Part model, mm, in its own coordinate system. A direction names the side the tool comes from. Give positions to 0.01 mm unless a question says otherwise; leave off trailing zeros. Order: outer loops, then holes, each group sorted by start corner. A loop starts at its lowest first (then second) coordinate and runs counter-clockwise, first axis right, second up. Notation, with made-up numbers: (23.25, 57.25) - (52.25, 57.25) arc R19 cw to (52.25, 66.25) - close; hole circle Ø9 at (70.5, -36.75). An arc over 180 degrees is marked (long way). One line per item, written item: value.
```python
from build123d import *

# Parameters (mm, degrees)
BASE_FLANGIA1_DEPTH       = 477.5
BORDO_FLANGIA1_DEPTH      = 436
BORDO_FLANGIA1_BEND_DEPTH = 436
TAGLIO_ESTRUSIONE2_START  = -275
TAGLIO_ESTRUSIONE2_DEPTH  = 550


# Read off the part's stored shape, not the designer's step: Taglio-Estrusione2
# Sheet-metal steps are written as plain solids
with BuildPart() as part:
    # Schizzo1 → Base-Flangia1 (new, symmetric)
    with BuildSketch(Plane.XY):
        with BuildLine():
            Line((-255, 50), (-228, 50))
            ThreePointArc((-228, 50), (-225.878679656, 49.121320344), (-225, 47))
            Line((-225, 47), (-225, 7))
            ThreePointArc((-225, 7), (-222.949747468, 2.050252532), (-218, 0))
            Line((-218, 0), (218, 0))
            ThreePointArc((218, 0), (222.949747468, 2.050252532), (225, 7))
            Line((225, 7), (225, 47))
            ThreePointArc((225, 47), (225.878679656, 49.121320344), (228, 50))
            Line((228, 50), (255, 50))
            Line((255, 50), (255, 54))
            Line((255, 54), (228, 54))
            ThreePointArc((228, 54), (223.050252532, 51.949747468), (221, 47))
            Line((221, 47), (221, 7))
            ThreePointArc((221, 7), (220.121320344, 4.878679656), (218, 4))
            Line((218, 4), (-218, 4))
            ThreePointArc((-218, 4), (-220.121320344, 4.878679656), (-221, 7))
            Line((-221, 7), (-221, 47))
            ThreePointArc((-221, 47), (-223.050252532, 51.949747468), (-228, 54))
            Line((-228, 54), (-255, 54))
            Line((-255, 54), (-255, 50))
        make_face()
    extrude(amount=BASE_FLANGIA1_DEPTH, both=True)

    # Bordo-Flangia1 section (across the edge) → Bordo-Flangia1 (add)
    with BuildSketch(Plane(origin=(-218, 4, 480.5), x_dir=(0, 0, -1), z_dir=(1, 0, 0))):
        with BuildLine():
            Line((-4, 3), (-4, 36))
            Line((-4, 36), (0, 36))
            Line((0, 36), (0, 3))
            ThreePointArc((0, 3), (0.878679656, 0.878679656), (3, 0))
            Line((3, 0), (3, -4))
            ThreePointArc((3, -4), (-1.949747468, -1.949747468), (-4, 3))
        make_face()
    extrude(amount=BORDO_FLANGIA1_DEPTH)

    # Bordo-Flangia1 section 2 (across the edge) → Bordo-Flangia1 bend (add)
    with BuildSketch(Plane(origin=(218, 4, -480.5), x_dir=(0, 0, 1), z_dir=(-1, 0, 0))):
        with BuildLine():
            Line((-4, 3), (-4, 36))
            Line((-4, 36), (0, 36))
            Line((0, 36), (0, 3))
            ThreePointArc((0, 3), (0.878679656, 0.878679656), (3, 0))
            Line((3, 0), (3, -4))
            ThreePointArc((3, -4), (-1.949747468, -1.949747468), (-4, 3))
        make_face()
    extrude(amount=BORDO_FLANGIA1_BEND_DEPTH)

    # Taglio-Estrusione2 outline → Taglio-Estrusione2 (cut)
    with BuildSketch(Plane.XY.offset(TAGLIO_ESTRUSIONE2_START)):
        with BuildLine():
            ThreePointArc((-228, 50), (-226.396432548, 49.535462765), (-225.289476291, 48.285714286))
            Line((-225.289476291, 48.285714286), (-221.67544468, 50))
            ThreePointArc((-221.67544468, 50), (-224.258342614, 52.916079783), (-228, 54))
            Line((-228, 54), (-255, 54))
            Line((-255, 54), (-255, 50))
            Line((-255, 50), (-228, 50))
        make_face()
        with BuildLine():
            ThreePointArc((228, 54), (224.258342614, 52.916079783), (221.67544468, 50))
            Line((221.67544468, 50), (225.289476291, 48.285714286))
            ThreePointArc((225.289476291, 48.285714286), (226.396432548, 49.535462765), (228, 50))
            Line((228, 50), (255, 50))
            Line((255, 50), (255, 54))
            Line((255, 54), (228, 54))
        make_face()
    extrude(amount=TAGLIO_ESTRUSIONE2_DEPTH, mode=Mode.SUBTRACT)


solid = part.part
```
1) Mould opens along Z. For faces 1 (the flat face through (-224, 35, -477.5)), 2 (the flat face through (242, 54, -375)), 3 (the flat face through (-3, 24, 480.5)) say: released by +Z, released by -Z, zero draft, split by the parting line, or undercut.
Outcome:
face 1: released by -Z
face 2: zero draft
face 3: undercut
2) Which spindle directions (+Z, -Z, +X, -X, +Y, -Y) get a long thin tool onto all of the face, cutting with end or side? Do faces 4 (the flat face through (221, 27, 7)), 5 (the flat face through (3, 24, -480.5)), 6 (the flat face through (3, 4, 7)). Say none if no direction does.
Outcome:
face 4: +Z, -Z, +Y
face 5: +X, -X, +Y
face 6: +Y
3) Drill centre lines: line 1 along Z through (x, y) = (20, 31); line 2 along X through (y, z) = (24.5, 92); line 3 along Y through (x, z) = (-129, -198). Where is each one in solid material? Low to high. Write a range as from..to.
Outcome:
line 1: z = -484.5..-480.5, 480.5..484.5
line 2: x = -225..-221, 221..225
line 3: y = 0..4
4) Pin check, flat tips, straight feed: pin 1 (8 mm diameter, centred on y = 39.5, z = 134, fed in from +X); pin 2 (13.5 mm diameter, centred on x = -243.5, z = -419.5, fed in from -Y); pin 3 (18.5 mm diameter, centred on x = 233, y = 27, fed in from -Z). Stop position of each tip, or through.
Outcome:
pin 1: stops at x = 225
pin 2: stops at y = 50
pin 3: stops at z = -477.5
5) Cut at C-C, the plane z = 148.5. Give the cut face in (x, y).
Outcome:
outline: (-225.29, 48.29) arc R3 cw to (-225, 47) - (-225, 7) arc R7 ccw to (-218, 0) - (218, 0) arc R7 ccw to (225, 7) - (225, 47) arc R3 cw to (225.29, 48.29) - (221.68, 50) arc R7 ccw to (221, 47) - (221, 7) arc R3 cw to (218, 4) - (-218, 4) arc R3 cw to (-221, 7) - (-221, 47) arc R7 ccw to (-221.68, 50) - close
6) Cut at A-A, the plane y = 25. Give the cut face in (x, z).
Outcome:
outline: (-225, -477.5) - (-221, -477.5) - (-221, 477.5) - (-225, 477.5) - close; (-218, -484.5) - (218, -484.5) - (218, -480.5) - (-218, -480.5) - close; (-218, 480.5) - (218, 480.5) - (218, 484.5) - (-218, 484.5) - close; (221, -477.5) - (225, -477.5) - (225, 477.5) - (221, 477.5) - close
7) Cut at B-B, the plane x = 171.5. Give the cut face in (y, z).
Outcome:
outline: (0, -477.5) arc R7 ccw to (7, -484.5) - (40, -484.5) - (40, -480.5) - (7, -480.5) arc R3 cw to (4, -477.5) - (4, 477.5) arc R3 cw to (7, 480.5) - (40, 480.5) - (40, 484.5) - (7, 484.5) arc R7 ccw to (0, 477.5) - close
